Part model, mm, in its own coordinate system. Face numbers are marked on the shaded views. Round coordinates to 2 decimals unless told otherwise and drop trailing zeros. Loops run counter-clockwise (first coordinate to the right, second up) from the corner with the lowest first, then second, coordinate; pieces in that order, holes last. Notation, with made-up numbers: M 18,36.25 L 43,36.25 A15 cw 43,63.25 Z; hole C 42,-12.75 d6. An arc over 180 degrees is marked long. Put each result on its own line as item: value. Start each with the question number.
1) Slice it at A-A on y = -3.5. Give the cut face in (x, z), then the cut area to 3 significant figures.
2) Probe line 1 along Z through (x, y) = (59.5, -45.9); line 2 along Y through (x, z) = (-75.5, 0.9); line 3 along Z through (x, y) = (59, -45). List the from-to ranges inside material, lowest first.
3) Drop flat-ended pins along their axis: pin 1 Ø2 at (x, z) = (59.5, 5.9) entering from -Y; pin 2 Ø11 at (x, y) = (-73, 24) entering from +Z; pin 3 Ø1.5 at (x, y) = (77.5, -4) entering from +Z. Give the stop position or say it passes through.
4) Pull direction Y, two halves, no side cores. Call the marked faces 1, 2 and 3: +Y half, -Y half, draft (parallel to the pull), parting line (faces both ways), or undercut.
Autodesk Fusion 360 part; units mm, degrees
sketch "Sketch1" plane through (0, 0, 0) normal (0, 0, 1) x (1, 0, 0)
  line L0 (-79.5, 48.75) -> (79.5, 48.75)
  line L1 (79.5, 48.75) -> (79.5, -48.75)
  line L2 (79.5, -48.75) -> (-79.5, -48.75)
  line L3 (-79.5, -48.75) -> (-79.5, 48.75)
  line L4 (-79.5, 0) -> (79.5, 0)
  dimension "d1" = 159
  dimension "d2" = 97.5
extrude "Extrude1" add sketch "Sketch1" along normal blind 30
sketch "Sketch2" plane through (-79.5, 0, 0) normal (-1, 0, 0) x (0, -1, 0)
  line L0 (-48.75, 0) -> (48.75, 0)
  line L1 (48.75, 0) -> (48.75, 30)
  line L2 (48.75, 30) -> (-48.75, 30)
  line L3 (-48.75, 30) -> (-48.75, 0)
  line L4 (-38, 23) -> (30, 23)
  line L5 (30, 23) -> (30, 6.5)
  line L6 (30, 6.5) -> (-38, 6.5)
  line L7 (-38, 6.5) -> (-38, 23)
  line L8 (-48.75, 30) -> (47.25, 30)
  line L9 (47.25, 30) -> (47.25, 1.5)
  line L10 (47.25, 1.5) -> (-48.75, 1.5)
  line L11 (-48.75, 1.5) -> (-48.75, 30)
  dimension "d5" = 68
  dimension "d6" = 16.5
  dimension "d7" = 10.75
  dimension "d8" = 6.5
  dimension "d9" = 1.5
  dimension "d10" = 1.5
extrude "Extrude2" cut sketch "Sketch2" against normal blind 10 contours L2 L3 L8 L9 L10 L11
extrude "Extrude3" add 1 faces at (-79.5, 15.3333, 17.5) along direction (-1, 0, 0) blind 5
sketch "Sketch3" plane through (79.5, 0, 0) normal (1, 0, 0) x (0, 1, 0)
  line L0 (-48.75, 0) -> (48.75, 0)
  line L1 (48.75, 0) -> (48.75, 30)
  line L2 (48.75, 30) -> (-48.75, 30)
  line L3 (-48.75, 30) -> (-48.75, 0)
  line L4 (-47.25, 30) -> (48.75, 30)
  line L5 (48.75, 30) -> (48.75, 4)
  line L6 (48.75, 4) -> (-47.25, 4)
  line L7 (-47.25, 4) -> (-47.25, 30)
  dimension "d15" = 1.5
  dimension "d16" = 4
extrude "Extrude4" cut sketch "Sketch3" against normal blind 5 contours L1 L2 L4 L5 L6 L7
sketch "Sketch4" plane through (0, 0, 4) normal (0, 0, 1) x (-1, 0, 0)
  line L0 (-79.5, 47.25) -> (-79.5, -48.75)
  line L1 (-79.5, -48.75) -> (-74.5, -48.75)
  line L2 (-74.5, -48.75) -> (-74.5, 47.25)
  line L3 (-74.5, 47.25) -> (-79.5, 47.25)
  line L4 (-79.5, 37.25) -> (-74.5, 37.25)
  dimension "d19" = 10
extrude "Extrude5" cut sketch "Sketch4" against normal blind 2.5 contours L0 L2 L3 L4
sketch "Sketch5" plane through (0, -48.75, 0) normal (0, -1, 0) x (1, 0, 0)
  line L0 (-79.5, 0) -> (79.5, 0)
  line L1 (79.5, 0) -> (79.5, 30)
  line L2 (79.5, 30) -> (-79.5, 30)
  line L3 (-79.5, 30) -> (-79.5, 0)
  circle A0 centre (-72.5, 26) radius 1.75
  circle A1 centre (76.9, 14.5) radius 1.75
  circle A2 centre (59.5, 23.9) radius 1.25
  circle A3 centre (59.5, 5.9) radius 1.25
  circle A4 centre (-57.5, 15) radius 1.25
  line L4 (76.9, 16.25) -> (79.5, 16.25)
  line L5 (76.9, 12.75) -> (79.5, 12.75)
  dimension "d22" = 2.5
  dimension "d23" = 2.5
  dimension "d24" = 3.5
  dimension "d25" = 2.6
  dimension "d26" = 14.5
  dimension "d27" = 18
  dimension "d28" = 20
  dimension "d29" = 5.9
  dimension "d30" = 20
  dimension "d31" = 137
  dimension "d32" = 15
  dimension "d33" = 3.5
  dimension "d34" = 26
  dimension "d35" = 152
  dimension "d36" = 2.5
extrude "Extrude6" cut sketch "Sketch5" against normal blind 13 contours A0
extrude "Extrude7" cut sketch "Sketch5" against normal blind 5 contours A4
extrude "Extrude8" cut sketch "Sketch5" against normal blind 1.5 contours L1 A1 L4 L5 | A1
extrude "Extrude9" cut sketch "Sketch5" against normal blind 5 contours A3
extrude "Extrude10" cut sketch "Sketch5" against normal blind 5 contours A2
sketch "Sketch6" plane through (0, 0, 0) normal (0, 0, -1) x (1, 0, 0)
  line L0 (79.5, 48.75) -> (-79.5, 48.75)
  line L1 (-79.5, 48.75) -> (-79.5, -48.75)
  line L2 (-79.5, -48.75) -> (79.5, -48.75)
  line L3 (79.5, -48.75) -> (79.5, 48.75)
  circle A0 centre (-75.5, -43.25) radius 1.75
  circle A1 centre (77.75, 42.05) radius 1.75
  line L4 (77.75, 43.8) -> (79.5, 43.8)
  line L5 (77.75, 40.3) -> (79.5, 40.3)
  dimension "d47" = 3.5
  dimension "d48" = 6.7
  dimension "d49" = 1.75
  dimension "d50" = 3.5
  dimension "d51" = 85.3
  dimension "d52" = 155
extrude "Extrude11" cut sketch "Sketch6" against normal blind 7 contours L3 A1 L4 | A1 | L3 A1 L5
extrude "Extrude12" cut sketch "Sketch6" against normal blind 1.5 contours A0
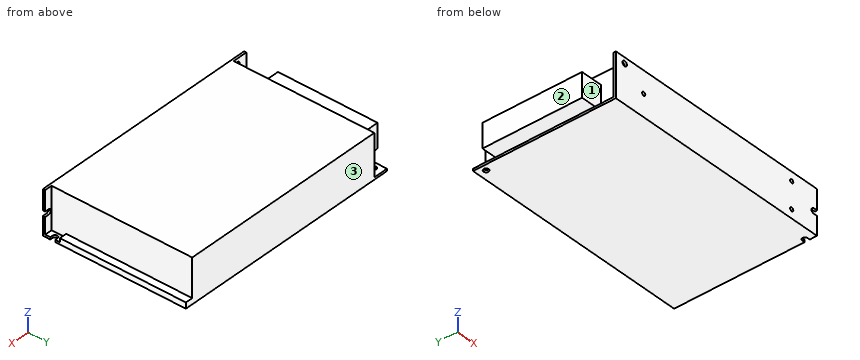
Recorded:
1. outline: M -84.5,6.5 L -69.5,6.5 L -69.5,1.5 L -79.5,1.5 L -79.5,0 L 79.5,0 L 79.5,4 L 74.5,4 L 74.5,30 L -69.5,30 L -69.5,23 L -84.5,23 Z
1. area: 4,600 mm2
2. line 1: z = 0 to 4.65, 7.15 to 22.65, 25.15 to 30
2. line 2: y = -48.75 to 41.5, 45 to 48.75
2. line 3: z = 0 to 4.75, 7.05 to 22.75, 25.05 to 30
3. pin 1: stops at y = -43.75
3. pin 2: stops at z = 30
3. pin 3: stops at z = 4
4. face 1: undercut
4. face 2: draft
4. face 3: +Y half
